Input: part model. Units: mm. Frame: model coordinates. Face numbers are marked on the shaded views. A direction names the side the tool comes from. Round coordinates to 2 decimals unless told otherwise and drop trailing zeros. Loops run counter-clockwise (first coordinate to the right, second up) from the corner with the lowest first, then second, coordinate; pieces in that order, holes last. Notation, with made-up numbers: (79.25, 16) - (107.25, 16) arc R34 ccw to (107.25, 51) - close; hole circle Ø2 at (-34, -26). An arc over 180 degrees is marked (long way). Write each question's results on one line, items separated by ' | '.
from build123d import *

# Parameters (mm, degrees)
F0_R     = 17.5
F0_R_2   = 5.05
F1_DEPTH = 4
F2_R     = 17.5
F3_DEPTH = 1
F4_SIZE  = 1
F5_SIZE  = 1


with BuildPart() as f1:
    # F0 (on Top) → F1 (new body)
    with BuildSketch(Plane.XY):
        Circle(F0_R)
        with Locations((-6.289302, -8.656482)):
            Circle(F0_R_2, mode=Mode.SUBTRACT)
        with Locations((6.289302, -8.656482)):
            Circle(F0_R_2, mode=Mode.SUBTRACT)
        with Locations((-10.176305, 3.306482)):
            Circle(F0_R_2, mode=Mode.SUBTRACT)
        Circle(F0_R_2, mode=Mode.SUBTRACT)
        with Locations((10.176305, 3.306482)):
            Circle(F0_R_2, mode=Mode.SUBTRACT)
        with Locations((0, 10.7)):
            Circle(F0_R_2, mode=Mode.SUBTRACT)
    extrude(amount=F1_DEPTH)

    # F2 (on face) → F3 (join)
    with BuildSketch(Plane.XY.offset(4)):
        Circle(F2_R)
    extrude(amount=F3_DEPTH)

    # F4
    f4_edges = [f1.edges().sort_by_distance(p)[0] for p in [
        (-17.5, 0, 0),
    ]]
    chamfer(f4_edges, length=F4_SIZE)

    # F5
    f5_edges = [f1.edges().sort_by_distance(p)[0] for p in [
        (-17.5, 0, 5),
    ]]
    chamfer(f5_edges, length=F5_SIZE)


solid = f1.part
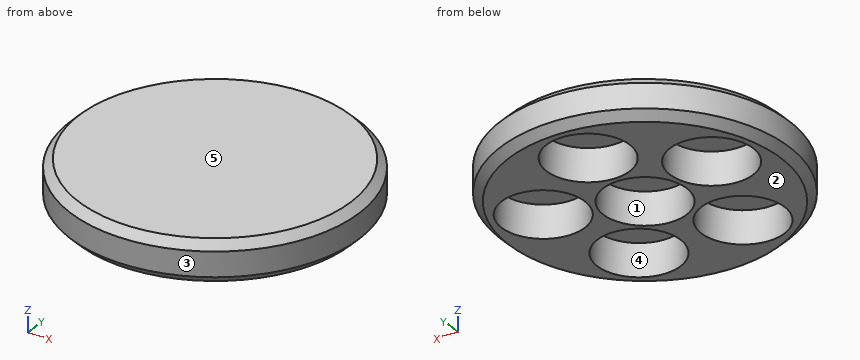
1. Section query C-C, the plane y = 0. Output: boundary loops of the cut face in (x, z).
Answer:
outline: (-17.5, 1) - (-16.5, 0) - (-13.99, 0) - (-13.99, 4) - (-6.36, 4) - (-6.36, 0) - (-5.05, 0) - (-5.05, 4) - (5.05, 4) - (5.05, 0) - (6.36, 0) - (6.36, 4) - (13.99, 4) - (13.99, 0) - (16.5, 0) - (17.5, 1) - (17.5, 4) - (16.5, 5) - (-16.5, 5) - (-17.5, 4) - close
2. Set-up query: the marked faces 4 and 5. Return all of +Z, -Z, +X, -X, +Y, -Y with unobstructed straight access to the full face (end or side cutting, diameter ignored); none if empty.
Answer:
face 4: -Z | face 5: +Z, +X, -X, +Y, -Y
3. Section query A-A, the plane x = 0. Output: boundary loops of the cut face in (y, z), plus the area to 3 significant figures.
Answer:
outline: (-17.5, 1) - (-16.5, 0) - (-5.05, 0) - (-5.05, 4) - (5.05, 4) - (5.05, 0) - (5.65, 0) - (5.65, 4) - (15.75, 4) - (15.75, 0) - (16.5, 0) - (17.5, 1) - (17.5, 4) - (16.5, 5) - (-16.5, 5) - (-17.5, 4) - close | area: 92.2 mm^2
4. Contact query for flat-ended pins moving along their axis: pin 1 (1.5 mm diameter, centred on x = -9, z = 0.5, fed in from +Y); pin 2 (8 mm diameter, centred on x = 6.29, y = -8.66, fed in from -Z). Output: stop coordinate, or through.
Answer:
pin 1: y = 15.33 | pin 2: z = 4
5. Mould query, pull axis Y, two halves, no side actions, for the marked faces 1, 2 and 3. Classes: pulls with the +Y half, pulls with the -Y half, needs draft (parallel to the pull), parting line crosses it, or undercut.
Answer:
face 1: undercut | face 2: needs draft | face 3: parting line crosses it
6. Section query B-B, the plane z = 2.95. Output: boundary loops of the cut face in (x, y).
Answer:
outline: circle Ø35 at (0, 0); hole circle Ø10.1 at (-10.18, 3.31); hole circle Ø10.1 at (-6.29, -8.66); hole circle Ø10.1 at (0, 0); hole circle Ø10.1 at (0, 10.7); hole circle Ø10.1 at (6.29, -8.66); hole circle Ø10.1 at (10.18, 3.31)
7. Line query: line 1 (Y direction, x = 0, z = 1.5); line 2 (Y direction, x = -3, z = 1.3); line 3 (Y direction, x = -4.5, z = 3.35). Output: solid intervals per line, ascending. Write a range as [from, to].
Answer:
line 1: [-17.5, -5.05], [5.05, 5.65], [15.75, 17.5] | line 2: [-17.24, -12.49], [-4.82, -4.06], [4.06, 6.64], [14.76, 17.24] | line 3: [-16.91, -13.38], [-3.93, -2.29], [2.29, 8.41], [12.99, 16.91]
